Design review of the part built by this model. Coordinates are the model's own, in mm. A direction names the side the tool comes from. Coordinates: 2 decimals unless noted, no trailing zeros. Write each loop counter-clockwise with the first axis right and the second up, starting at its lowest first coordinate (ties: lowest second). Pieces come first, ordered by that corner, then holes.
Q1. Take a section at B-B (y = 8). Give the boundary of the cut face in (x, z).
Q2. Take a section at D-D (y = 24.25). Give the boundary of the cut face in (x, z).
Q3. Take a section at C-C (z = 12). Give the boundary of the cut face in (x, y), and give its area (3 significant figures).
Q4. Take a section at A-A (x = 25). Give the boundary of the cut face in (y, z), and give its area (3 significant figures).
Q5. For probe 1 along X at (y, z) = (16.5, -16); probe 2 along Y at (x, z) = (8, -19.5); probe 3 along X at (y, z) = (16.75, 1), list the stretches that pass through material, from the lowest coordinate up.
Q6. Mouldability with a two-part tool opening along Z and no side actions: class faces 5 (the flat face through (38.438, -0.493, 8.968)), 6 (the flat face through (38.023, 19, 7)), 7 (the flat face through (-38, 19, -16.842)), 8 (the cylindrical face through (33.01, 13.436, -29.816)) as pulls with the +Z half, pulls with the -Z half, needs draft (parallel to the pull), parting line crosses it, or undercut.
Q7. Insertion check: pin 1 (1 mm diameter, centred on x = 32.5, y = 21, fed in from +Z); pin 2 (2 mm diameter, centred on y = 20, z = -20, fed in from -X); pin 3 (2 mm diameter, centred on y = 8, z = -22, fed in from +X); pin 4 (4 mm diameter, centred on y = 20.5, z = 9.5, fed in from -X). Each pin has a flat end and moves straight along its axis. Give the tip position at first contact, or say it passes through.
Q8. Machinability: for faces 1 (the flat face through (38.28, -0.49, -18.16)), 2 (the cylindrical face through (35.843, 13.055, 9.053)), 3 (the flat face through (-33.833, -0.493, -18.158)), 4 (the cylindrical face through (-31.397, 17.548, -23.542)), which of the approach directions +Z, -Z, +X, -X, +Y, -Y give a long, thin tool a straight path to every point of the face, cutting with its end or side? Answer none if there is none.
```python
from build123d import *

# Parameters (mm, degrees)
SZKIC1_W                    = 63
SZKIC1_H                    = 52
DODANIE_WYCI_GNI_CIE1_DEPTH = 29
ZAOKR_GLENIE1_R             = 2.5
DODANIE_WYCI_GNI_CIE2_DEPTH = 1
SZKIC3_R                    = 2.45
WYTNIJ_WYCI_GNI_CIE6_DEPTH  = 62.065626678
SZKIC4_R                    = 6.5
DODANIE_WYCI_GNI_CIE3_DEPTH = 4.3
SZKIC5_W                    = 1
SZKIC5_H                    = 6.5
DODANIE_WYCI_GNI_CIE4_DEPTH = 9
LUSTRO4_COPY_1_SKETCH_W     = 1
LUSTRO4_COPY_1_SKETCH_H     = 6.5
LUSTRO4_COPY_1_DEPTH        = 9
LUSTRO4_COPY_2_SKETCH_W     = 1
LUSTRO4_COPY_2_SKETCH_H     = 6.5
LUSTRO4_COPY_2_DEPTH        = 9


with BuildPart() as part:
    # Szkic1 → Dodanie-wyciągnięcie1 (new body)
    with BuildSketch(Plane(origin=(0, 0, 0), x_dir=(1, 0, 0), z_dir=(0, 1, 0))):
        with Locations((2.222834646, 4.567716535)):
            Rectangle(SZKIC1_W, SZKIC1_H)
    extrude(amount=DODANIE_WYCI_GNI_CIE1_DEPTH)

    # Zaokrąglenie1
    zaokr_glenie1_edges = [part.edges().sort_by_distance(p)[0] for p in [
        (33.722834646, 29, -4.567716535),
        (2.222834646, 29, -30.567716535),
        (-29.277165354, 29, -4.567716535),
        (2.222834646, 29, 21.432283465),
        (-29.277165354, 14.5, -30.567716535),
        (33.722834646, 14.5, -30.567716535),
        (33.722834646, 14.5, 21.432283465),
        (-29.277165354, 14.5, 21.432283465),
    ]]
    fillet(zaokr_glenie1_edges, radius=ZAOKR_GLENIE1_R)

    # Szkic2 → Dodanie-wyciągnięcie2 (add)
    with BuildSketch(Plane.XZ):
        with BuildLine():
            Line((-39.289158378, -2.43984114), (-28.544932307, 20.700050418))
            Line((-28.544932307, 20.700050418), (-28.544932307, -29.312606034))
            Line((-28.544932307, -29.312606034), (-39.272080362, -6.687578711))
            ThreePointArc((-39.272080362, -6.687578711), (-39.754125902, -4.565613657), (-39.289158378, -2.43984114))
        make_face()
        with BuildLine():
            Line((32.990601599, 20.700050418), (32.990601599, -29.312606034))
            Line((32.990601599, -29.312606034), (43.717749653, -6.687578711))
            ThreePointArc((43.717749653, -6.687578711), (44.199795194, -4.565613657), (43.734827669, -2.43984114))
            Line((43.734827669, -2.43984114), (32.990601599, 20.700050418))
        make_face()
    extrude(amount=DODANIE_WYCI_GNI_CIE2_DEPTH)

    # Szkic3 → Wytnij-wyciągnięcie6 (cut, through all)
    with BuildSketch(Plane.XZ):
        with Locations(Location((-35.027165354, -4.306277808, 0), (0, 0, 270))):
            Circle(SZKIC3_R)
        with Locations(Location((39.472834646, -4.306277808, 0), (0, 0, 90))):
            Circle(SZKIC3_R)
    extrude(amount=WYTNIJ_WYCI_GNI_CIE6_DEPTH, mode=Mode.SUBTRACT)

    # Szkic4 → Dodanie-wyciągnięcie3 (add)
    with BuildSketch(Plane.ZY.offset(29.277165354)):
        with Locations(Location((8.206789605, 19.5, 0), (0, 0, 180))):
            Circle(SZKIC4_R)
        with Locations(Location((-17.342222675, 19.5, 0), (0, 0, 180))):
            Circle(SZKIC4_R)
    dodanie_wyci_gni_cie3 = extrude(amount=DODANIE_WYCI_GNI_CIE3_DEPTH)

    # Szkic5 → Dodanie-wyciągnięcie4 (add)
    with BuildSketch(Plane.ZY.offset(33.577165354)):
        with Locations((8.206789605, 19.5)):
            Rectangle(SZKIC5_W, SZKIC5_H)
    dodanie_wyci_gni_cie4 = extrude(amount=DODANIE_WYCI_GNI_CIE4_DEPTH)

    # Lustro1: Dodanie-wyciągnięcie4 across plane
    add(dodanie_wyci_gni_cie4.mirror(Plane(origin=(0, 0, -4.567716535), x_dir=(1, 0, 0), z_dir=(0, 0, -1))))

    # Lustro2: Dodanie-wyciągnięcie3 across plane
    add(dodanie_wyci_gni_cie3.mirror(Plane.ZY.offset(-2.222834646)))

    # Lustro3: Dodanie-wyciągnięcie4 across plane
    add(dodanie_wyci_gni_cie4.mirror(Plane.ZY.offset(-2.222834646)))

    # Lustro4 copy 1 sketch → Lustro4 copy 1 (add)
    with BuildSketch(Plane(origin=(38.022834646, 0, -9.135433071), x_dir=(0, 0, -1), z_dir=(1, 0, 0))):
        with Locations((8.206789605, 19.5)):
            Rectangle(LUSTRO4_COPY_1_SKETCH_W, LUSTRO4_COPY_1_SKETCH_H)
    extrude(amount=LUSTRO4_COPY_1_DEPTH)

    # Lustro4 copy 2 sketch → Lustro4 copy 2 (add)
    with BuildSketch(Plane(origin=(38.022834646, 0, 0), x_dir=(0, 0, 1), z_dir=(1, 0, 0))):
        with Locations((8.206789605, -19.5)):
            Rectangle(LUSTRO4_COPY_2_SKETCH_W, LUSTRO4_COPY_2_SKETCH_H)
    extrude(amount=LUSTRO4_COPY_2_DEPTH)


solid = part.part
```
Response:
1. outline: (-29.28, -28.07) arc R2.5 ccw to (-26.78, -30.57) - (31.22, -30.57) arc R2.5 ccw to (33.72, -28.07) - (33.72, 18.93) arc R2.5 ccw to (31.22, 21.43) - (-26.78, 21.43) arc R2.5 ccw to (-29.28, 18.93) - close
2. outline: (-33.58, -21.78) - (-29.28, -21.78) - (-29.28, -28.07) arc R2.5 ccw to (-26.78, -30.57) - (31.22, -30.57) arc R2.5 ccw to (33.72, -28.07) - (33.72, -21.78) - (38.02, -21.78) - (38.02, -12.91) - (33.72, -12.91) - (33.72, 3.77) - (38.02, 3.77) - (38.02, 12.64) - (33.72, 12.64) - (33.72, 18.93) arc R2.5 ccw to (31.22, 21.43) - (-26.78, 21.43) arc R2.5 ccw to (-29.28, 18.93) - (-29.28, 12.64) - (-33.58, 12.64) - (-33.58, 3.77) - (-29.28, 3.77) - (-29.28, -12.91) - (-33.58, -12.91) - close
3. outline: (-33.58, 14.22) - (-29.28, 14.22) - (-29.28, 0) - (-32.58, 0) - (-32.58, -1) - (-28.54, -1) - (-28.54, 0) - (32.99, 0) - (32.99, -1) - (37.03, -1) - (37.03, 0) - (33.72, 0) - (33.72, 14.22) - (38.02, 14.22) - (38.02, 24.78) - (33.72, 24.78) - (33.72, 26.5) arc R2.5 ccw to (31.22, 29) - (-26.78, 29) arc R2.5 ccw to (-29.28, 26.5) - (-29.28, 24.78) - (-33.58, 24.78) - close
3. area: 1,920 mm2
4. outline: (0, -30.57) - (26.5, -30.57) arc R2.5 ccw to (29, -28.07) - (29, 18.93) arc R2.5 ccw to (26.5, 21.43) - (0, 21.43) - close
4. area: 1,510 mm2
5. probe 1: x = -33.58 to 38.02
5. probe 2: y = 0 to 29
5. probe 3: x = -29.28 to 33.72
6. face 5: pulls with the +Z half
6. face 6: undercut
6. face 7: undercut
6. face 8: pulls with the -Z half
7. pin 1: stops at z = 21.31
7. pin 2: stops at x = -33.58
7. pin 3: stops at x = 33.72
7. pin 4: stops at x = -42.58
8. face 1: -Z, +X, -Y
8. face 2: +X
8. face 3: -Z, -X, -Y
8. face 4: -X
